from build123d import *

# Parameters (mm, degrees)
F1_DEPTH = 50


with BuildPart() as f1:
    # F0 (on Front) → F1 (new body)
    with BuildSketch(Plane.XZ):
        Polygon((-35.267115, 11.45898), (-21.796276, -30), (21.796276, -30), (35.267115, 11.45898), (0, 37.082039), align=None)
        Polygon((-16.933772, 0.669846), (-8.466886, 15.334923), (8.466886, 15.334923), (16.933772, 0.669846), (8.466886, -13.995231), (-8.466886, -13.995231), align=None, mode=Mode.SUBTRACT)
    extrude(amount=F1_DEPTH)


solid = f1.part
The listing builds one solid part. Answer for the finished solid, in the listing's coordinates (mm). A direction names the side the tool comes from. Round coordinates to 2 decimals unless told otherwise and drop trailing zeros. Order: outer loops, then holes, each group sorted by start corner. A loop starts at its lowest first (then second) coordinate and runs counter-clockwise, first axis right, second up. Notation, with made-up numbers: (25, -29) - (47, -29) arc R19 cw to (47, 1) - close; hole circle Ø3 at (72.5, -1.5). An arc over 180 degrees is marked (long way). Write item = value, one per line. Start each with the question number.
1) For a pull along X with two mould halves and no side action, classify faces 3 (the flat face through (15, 0, -3)), 4 (the flat face through (-28.626, -24.65, -8.98)), 5 (the flat face through (12.64, -24.65, 8.11)) as released by +X, released by -X, zero draft, split by the parting line, or undercut.
2) Section A-A, the plane x = -2 is taken. Write down the section's boundary in (y, z), plus the area to 3 significant figures.
3) Section D-D, the plane x = 26 is taken. Write down the section's boundary in (y, z), plus the area to 3 significant figures.
4) Straight lines are drawn through the part: L1, parallel to Z at x = -15, y = -42; L2, parallel to X at y = -30.5, z = 5; L3, parallel to X at y = -9.5, z = 15. For each, find the intervals that lie inside material, in ascending order.
5) Section C-C, the plane z = 13.5 is taken. Write down the section's boundary in (x, y), plus the area to 3 significant figures.
6) Given pin 1 (12 mm diameter, centred on y = -29.5, z = 25.5, fed in from -X); pin 2 (1.5 mm diameter, centred on y = -20, z = 2.5, fed in from +X); pin 3 (4 mm diameter, centred on y = -28.5, z = 23, fed in from -X) (3 decimals), each flat-ended and moving along its own axis, determine where each tip first touches the part or whether it passes through.
7) For faces 1 (the flat face through (28.437, -24.65, -9.561)), 2 (the flat face through (0, -25, 15.335)), determine the directions among +Z, -Z, +X, -X, +Y, -Y from which every point of the face is accessible in a straight line to the end or side of a thin tool.
8) Section B-B, the plane y = -46 is taken. Write down the section's boundary in (x, z), plus the area to 3 significant figures.
Results list:
q1.face_3 = zero draft
q1.face_4 = released by -X
q1.face_5 = undercut
q2.outline = (-50, -30) - (0, -30) - (0, -14) - (-50, -14) - close; (-50, 15.33) - (0, 15.33) - (0, 35.63) - (-50, 35.63) - close
q2.area = 1,810 mm^2
q3.outline = (-50, -17.06) - (0, -17.06) - (0, 18.19) - (-50, 18.19) - close
q3.area = 1,760 mm^2
q4.L1 = -30 to -2.68, 4.02 to 26.18
q4.L2 = -33.17 to -14.43, 14.43 to 33.17
q4.L3 = -30.39 to -8.66, 8.66 to 30.39
q5.outline = (-32.46, -50) - (-9.53, -50) - (-9.53, 0) - (-32.46, 0) - close; (9.53, -50) - (32.46, -50) - (32.46, 0) - (9.53, 0) - close
q5.area = 2,290 mm^2
q6.pin_1 = -24.2
q6.pin_2 = 32.6
q6.pin_3 = -22.135
q7.face_1 = -Z, +X, +Y, -Y
q7.face_2 = +Y, -Y
q8.outline = (-35.27, 11.46) - (-21.8, -30) - (21.8, -30) - (35.27, 11.46) - (0, 37.08) - close; hole (-16.93, 0.67) - (-8.47, -14) - (8.47, -14) - (16.93, 0.67) - (8.47, 15.33) - (-8.47, 15.33) - close
q8.area = 2,520 mm^2
